Build history of the part. All positions in model axes, mm. A direction names the side the tool comes from. Round coordinates to 2 decimals unless told otherwise and drop trailing zeros. Write each loop counter-clockwise with the first axis right and the second up, starting at its lowest first coordinate (ties: lowest second). Pieces come first, ordered by that corner, then holes. Notation, with made-up numbers: M 3,23.5 L 59,23.5 A19 cw 59,47.5 Z; hole C -33.75,64.25 d6. An arc over 180 degrees is marked long. Write item = value, one per line. Start each with the question number.
Q1. Probe L1, parallel to Y at x = 0, z = 287.5; L2, parallel to Z at x = 59, y = -50; L3, parallel to Y at x = 62, z = 337.5. List the from-to ranges inside material, lowest first.
Q2. Band-saw the part on C-C on z = 501.5. Write the cut outline in (x, y).
Q3. Pull direction X, two halves, no side cores. Call faces 1 (the flat face through (33, -60, 250)), 2 (the flat face through (-1, 1, 571)), 3 (the flat face through (-119, -115, 269)), 4 (the cylindrical face through (-103.46, -42.9, 161.92)): released by +X, released by -X, zero draft, split by the parting line, or undercut.
Q4. Drop flat-ended pins along their axis: P1, Ø2.5, axis at x = -118, z = 260, coming from the -Y side; P2, Ø6, axis at x = 22, y = -198, coming from the -Z side; P3, Ø1.5, axis at x = 96, z = 203, coming from the +Y side. Give the stop position or say it passes through.
Q5. Band-saw the part on A-A on y = -153. Write the cut outline in (x, z).
Q6. Band-saw the part on D-D on y = -441.5. Write the cut outline in (x, z).
Q7. Tool access for faces 5 (the cylindrical face through (-39.997, 62.734, 311.347)), 6 (the flat face through (-110, -53, 169)), 7 (the cylindrical face through (-255.334, -302.056, 272.99)), 8 (the flat face through (-116, -115, 269)): list every direction of +Z, -Z, +X, -X, +Y, -Y with a clear straight run to the whole face (end or side of a thin tool).
Q8. Band-saw the part on B-B on x = 0. Write the cut outline in (y, z).
```python
from build123d import *

# Parameters (mm, degrees)
F2_R      = 68
F3_DEPTH  = 500
F1_FACE_R = 68.2
F4_DEPTH  = 200
F5_W      = 3
F5_H      = 250
F6_DEPTH  = 375


with BuildPart() as f1:
    # F0 (on Front) → F1 (revolve)
    with BuildSketch(Plane.XZ):
        Polygon((-255.4, 169), (-114, 169), (-112, 168), (-112, 156), (0, 156), (0, 371), (-68.2, 371), (-68.2, 250), (-74.4, 250), (-74.4, 371), (-255.4, 371), align=None)
    revolve(axis=Axis((0, 0, 263.5), (0, 0, -1)))

    # F2 (on Front) → F3 (join)
    with BuildSketch(Plane.XZ):
        with Locations((-187.4, 270)):
            Circle(F2_R)
    extrude(amount=F3_DEPTH)

    # F1_face (on face) → F4 (join)
    with BuildSketch(Plane.XY.offset(371)):
        Circle(F1_FACE_R)
    extrude(amount=F4_DEPTH)

    # F5 (on Top) → F6 (cut)
    with BuildSketch(Plane.XY):
        with Locations((-117.5, -125)):
            Rectangle(F5_W, F5_H)
    extrude(amount=F6_DEPTH, mode=Mode.SUBTRACT)


solid = f1.part
```
Conclusion:
q1.L1 = -255.4 to -74.4, -68.2 to 68.2, 74.4 to 255.4
q1.L2 = 156 to 371
q1.L3 = -247.76 to -41.13, -28.41 to 28.41, 41.13 to 247.76
q2.outline = C 0,0 d136.4
q3.face_1 = undercut
q3.face_2 = zero draft
q3.face_3 = undercut
q3.face_4 = split by the parting line
q4.P1 = -225.98
q4.P2 = 169
q4.P3 = 236.97
q5.outline = M -204.5,169 L -119,169 L -119,371 L -204.5,371 L -204.5,335.81 A68 ccw -204.5,204.19 Z; M -116,169 L 204.5,169 L 204.5,371 L -116,371 Z
q6.outline = C -187.4,270 d136
q7.face_5 = +Z
q7.face_6 = -Z
q7.face_7 = -Y
q7.face_8 = +Z, -Z, -Y
q8.outline = M -255.4,169 L -114,169 L -112,168 L -112,156 L 112,156 L 112,168 L 114,169 L 255.4,169 L 255.4,371 L 74.4,371 L 74.4,250 L 68.2,250 L 68.2,571 L -68.2,571 L -68.2,250 L -74.4,250 L -74.4,371 L -255.4,371 Z
